Read the model definition and answer for the solid it produces. Units are mm, in the model's axes. Round coordinates to 2 decimals unless told otherwise and drop trailing zeros. Loops run counter-clockwise (first coordinate to the right, second up) from the corner with the lowest first, then second, coordinate; pieces in that order, holes last. Notation, with made-up numbers: M 34,26 L 71,26 A30 cw 71,57 Z; hole C 2.5,52.5 d5. An arc over 180 degrees is marked long. Write each question's results on one line, items separated by ' | '.
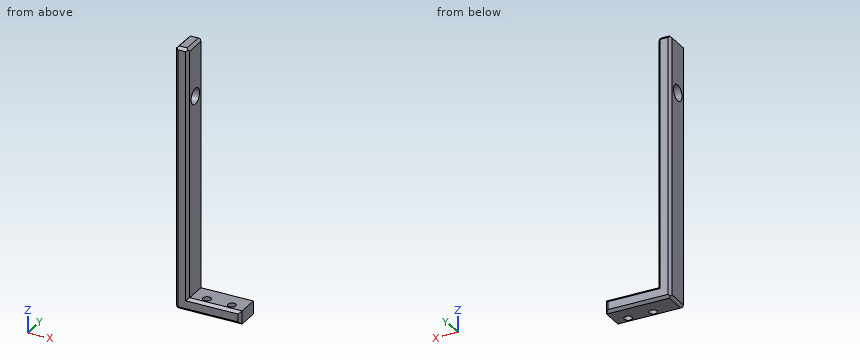
from build123d import *

# Parameters (mm, degrees)
BOSS_EXTRUDE1_DEPTH = 10
SKETCH2_R           = 3
CUT_EXTRUDE1_DEPTH  = 10
SKETCH3_R           = 1.5
CUT_EXTRUDE2_DEPTH  = 20
CHAMFER1_SIZE       = 1
CHAMFER2_SIZE       = 1
CHAMFER3_SIZE       = 1
CHAMFER4_SIZE       = 1


with BuildPart() as part:
    # Sketch1 → Boss-Extrude1 (new body)
    with BuildSketch(Plane(origin=(0, 0, 0), x_dir=(1, 0, 0), z_dir=(0, 1, 0))):
        Polygon((0, 0), (0, 100), (25, 100), (25, 95), (5, 95), (5, 0), align=None)
    extrude(amount=BOSS_EXTRUDE1_DEPTH)

    # Sketch2 → Cut-Extrude1 (cut)
    with BuildSketch(Plane(origin=(0, 0, 0), x_dir=(0, 0, -1), z_dir=(1, 0, 0))):
        with Locations((20.069491085, 5)):
            Circle(SKETCH2_R)
    extrude(amount=CUT_EXTRUDE1_DEPTH, mode=Mode.SUBTRACT)

    # Sketch3 → Cut-Extrude2 (cut)
    with BuildSketch(Plane(origin=(0, 0, -100), x_dir=(-1, 0, 0), z_dir=(0, 0, -1))):
        with Locations((-20, 3)):
            Circle(SKETCH3_R)
        with Locations((-10.5, 3)):
            Circle(SKETCH3_R)
    extrude(amount=-CUT_EXTRUDE2_DEPTH, mode=Mode.SUBTRACT)

    # Chamfer1
    chamfer1_edges = [part.edges().sort_by_distance(p)[0] for p in [
        (15, 10, -95),
        (25, 10, -97.5),
        (12.5, 10, -100),
        (0, 10, -50),
        (2.5, 10, 0),
        (5, 10, -47.5),
    ]]
    chamfer(chamfer1_edges, length=CHAMFER1_SIZE)

    # Chamfer2
    chamfer2_edges = [part.edges().sort_by_distance(p)[0] for p in [
        (0, 0, -50),
        (12.5, 0, -100),
        (25, 0, -97.5),
        (15, 0, -95),
        (5, 0, -47.5),
        (2.5, 0, 0),
    ]]
    chamfer(chamfer2_edges, length=CHAMFER2_SIZE)

    # Chamfer3
    chamfer3_edges = [part.edges().sort_by_distance(p)[0] for p in [
        (0, 5, -100),
    ]]
    chamfer(chamfer3_edges, length=CHAMFER3_SIZE)

    # Chamfer4
    chamfer4_edges = [part.edges().sort_by_distance(p)[0] for p in [
        (0, 5, 0),
        (5, 5, 0),
    ]]
    chamfer(chamfer4_edges, length=CHAMFER4_SIZE)


solid = part.part
Item 1: The part is cut by section A-A (x = 10.5). Determine the outline of the cut face in (y, z), plus the area to 3 significant figures.
Outcome:
outline: M 0,-99 L 1,-100 L 1.5,-100 L 1.5,-95 L 1,-95 L 0,-96 Z; M 4.5,-100 L 9,-100 L 10,-99 L 10,-96 L 9,-95 L 4.5,-95 Z | area: 33.0 mm2
Item 2: The part is cut by section D-D (z = -60). Determine the outline of the cut face in (x, y), plus the area to 3 significant figures.
Outcome:
outline: M 0,1 L 1,0 L 4,0 L 5,1 L 5,9 L 4,10 L 1,10 L 0,9 Z | area: 48.0 mm2
Item 3: The part is cut by section C-C (x = 17.5). Determine the outline of the cut face in (y, z).
Outcome:
outline: M 0,-99 L 1,-100 L 9,-100 L 10,-99 L 10,-96 L 9,-95 L 1,-95 L 0,-96 Z
Item 4: Flat-ended cylindrical pins translate along their axes: pin 1 (4 mm diameter, centred on y = 3.5, z = -63, fed in from +X); pin 2 (5 mm diameter, centred on x = 20, y = 3, fed in from +Z); pin 3 (2.5 mm diameter, centred on x = 10.5, y = 3, fed in from -Z). Find the tip coordinate at first contact, or state that the pin passes through.
Outcome:
pin 1: stops at x = 5 | pin 2: stops at z = -95 | pin 3: passes through
Item 5: Straight lines are drawn through the part: line 1 (Y direction, x = 10.5, z = -98.25); line 2 (Z direction, x = 2.8, y = 5); line 3 (X direction, y = 5.25, z = -61). For each, find the intervals that lie inside material, in ascending order.
Outcome:
line 1: y = 0 to 1.5, 4.5 to 10 | line 2: z = -100 to -23.07, -17.07 to 0 | line 3: x = 0 to 5
Item 6: The part is cut by section B-B (y = 6.5). Determine the outline of the cut face in (x, z), plus the area to 3 significant figures.
Outcome:
outline: M 0,-99 L 1,-100 L 25,-100 L 25,-95 L 5,-95 L 5,-22.67 L 0,-22.67 Z; M 0,-17.47 L 5,-17.47 L 5,-1 L 4,0 L 1,0 L 0,-1 Z | area: 573 mm2
